The model under review builds one solid part; all positions refer to its coordinate system, in mm. A direction names the side the tool comes from. Give positions to 0.01 mm unless a question says otherwise; leave off trailing zeros. Order: outer loops, then holes, each group sorted by start corner. A loop starts at its lowest first (then second) coordinate and runs counter-clockwise, first axis right, second up. Notation, with made-up numbers: (70, 62) -> (98, 62) arc R19 cw to (98, 87) -> close; hole circle Ø2 at (11.25, 22.25). An arc over 180 degrees is marked (long way). Answer as a JSON object with one key per item and string values. Group by question number.
from build123d import *

# Parameters (mm, degrees)
SKETCH_R        = 2.6
PAD_DEPTH       = 12
SKETCH001_W     = 20
SKETCH001_H     = 20
POCKET_DEPTH    = 5
SKETCH002_R     = 4.5
POCKET001_DEPTH = 12
SKETCH003_R     = 10.85
POCKET002_DEPTH = 8
SKETCH004_R     = 5.95
POCKET003_DEPTH = 4
SKETCH005_R     = 1.5
POCKET004_DEPTH = 19
SKETCH006_R     = 2.811214
POCKET005_DEPTH = 4
SKETCH007_R     = 4
POCKET006_DEPTH = 3
SKETCH008_R     = 1.5
POCKET007_DEPTH = 16
SKETCH009_R     = 1.5
POCKET008_DEPTH = 16


with BuildPart() as part:
    # Sketch → Pad (new body)
    with BuildSketch(Plane.XY):
        with BuildLine():
            Line((-57.237457, 55.978201), (32.762543, 55.978201))
            Line((32.762543, 55.978201), (32.762543, 25.978201))
            Line((32.762543, 25.978201), (35.725993, 25.978201))
            ThreePointArc((37.762543, 23.941651), (37.166051, 25.381709), (35.725993, 25.978201))
            Line((37.762543, 23.941651), (37.762543, 20.978201))
            Line((37.762543, -6.948806), (37.762543, 20.978201))
            Line((8.727398, -6.948806), (37.762543, -6.948806))
            ThreePointArc((6.368817, -5.446224), (7.329126, -6.541247), (8.727398, -6.948806))
            Line((-1.496911, 11.421883), (6.368817, -5.446224))
            ThreePointArc((-1.496911, 11.421883), (-2.47295, 12.534842), (-3.894125, 12.949077))
            Line((-20.852174, 12.949077), (-3.894125, 12.949077))
            ThreePointArc((-20.852174, 12.949077), (-22.12751, 12.577351), (-23.003388, 11.578602))
            Line((-31.391573, -6.409918), (-23.003388, 11.578602))
            ThreePointArc((-32.237457, -6.948806), (-31.73598, -6.802638), (-31.391573, -6.409918))
            Line((-62.237457, -6.948806), (-32.237457, -6.948806))
            Line((-62.237457, 17.407665), (-62.237457, -6.948806))
            Line((-62.237457, 17.407665), (-62.237457, 24.590235))
            ThreePointArc((-60.849491, 25.978201), (-61.830931, 25.571675), (-62.237457, 24.590235))
            Line((-60.849491, 25.978201), (-57.237457, 25.978201))
            Line((-57.237457, 25.978201), (-57.237457, 55.978201))
        make_face()
        with Locations((-49.737457, 6.02373)):
            Circle(SKETCH_R, mode=Mode.SUBTRACT)
        with Locations((-31.737457, 6.02373)):
            Circle(SKETCH_R, mode=Mode.SUBTRACT)
        with Locations((25.262543, 5.551194)):
            Circle(SKETCH_R, mode=Mode.SUBTRACT)
        with Locations((7.262543, 5.551194)):
            Circle(SKETCH_R, mode=Mode.SUBTRACT)
    extrude(amount=PAD_DEPTH)

    # Sketch001 (on Face26 of Pad) → Pocket (cut)
    with BuildSketch(Plane.XY.offset(12)):
        with Locations((-49.737457, 6.02373)):
            Rectangle(SKETCH001_W, SKETCH001_H)
        with Locations((25.262543, 5.551194)):
            Rectangle(SKETCH001_W, SKETCH001_H)
    extrude(amount=-POCKET_DEPTH, mode=Mode.SUBTRACT)

    # Sketch002 (on Face5 of Pocket) → Pocket001 (cut)
    with BuildSketch(Plane.XY.offset(12)):
        with Locations((-12.237457, 40.978201)):
            Circle(SKETCH002_R)
    extrude(amount=-POCKET001_DEPTH, mode=Mode.SUBTRACT)

    # Sketch003 (on Face5 of Pocket001) → Pocket002 (cut)
    with BuildSketch(Plane.XY.offset(12)):
        with Locations((-12.237457, 40.978201)):
            Circle(SKETCH003_R)
    extrude(amount=-POCKET002_DEPTH, mode=Mode.SUBTRACT)

    # Sketch004 (on Face5 of Pocket002) → Pocket003 (cut)
    with BuildSketch(Plane.XY.offset(12)):
        with Locations((-36.737457, 40.978201)):
            Circle(SKETCH004_R)
        with Locations((12.262543, 40.978201)):
            Circle(SKETCH004_R)
    extrude(amount=-POCKET003_DEPTH, mode=Mode.SUBTRACT)

    # Sketch005 (on Face18 of Pocket003) → Pocket004 (cut)
    with BuildSketch(Plane.XZ.offset(-12.949077)):
        with Locations((-12.237457, 8)):
            Circle(SKETCH005_R)
    extrude(amount=-POCKET004_DEPTH, mode=Mode.SUBTRACT)

    # Sketch006 (on Face18 of Pocket004) → Pocket005 (cut)
    with BuildSketch(Plane.XZ.offset(-12.949077)):
        with Locations((-12.237457, 8)):
            Circle(SKETCH006_R)
    extrude(amount=-POCKET005_DEPTH, mode=Mode.SUBTRACT)

    # Sketch007 (on Face4 of Pocket005) → Pocket006 (cut)
    with BuildSketch(Plane(origin=(0, 0, 0), x_dir=(1, 0, 0), z_dir=(0, 0, -1))):
        with Locations((-49.737457, -6.02373)):
            Circle(SKETCH007_R)
        with Locations((-31.737457, -6.02373)):
            Circle(SKETCH007_R)
        with Locations((7.262543, -5.551194)):
            Circle(SKETCH007_R)
        with Locations((25.262543, -5.551194)):
            Circle(SKETCH007_R)
    extrude(amount=-POCKET006_DEPTH, mode=Mode.SUBTRACT)

    # Sketch008 (on Face9 of Pocket006) → Pocket007 (cut)
    with BuildSketch(Plane.YZ.offset(32.762543)):
        with Locations((40.978201, 10)):
            Circle(SKETCH008_R)
    extrude(amount=-POCKET007_DEPTH, mode=Mode.SUBTRACT)

    # Sketch009 (on Face3 of Pocket007) → Pocket008 (cut)
    with BuildSketch(Plane(origin=(-57.237457, 0, 0), x_dir=(0, -1, 0), z_dir=(-1, 0, 0))):
        with Locations((-40.978201, 10)):
            Circle(SKETCH009_R)
    extrude(amount=-POCKET008_DEPTH, mode=Mode.SUBTRACT)


solid = part.part
1. Take a section at A-A on x = 25. Give the boundary of the cut face in (y, z), plus the area to 3 significant figures.
2. Machinability: for faces 3 (the flat face through (27, 8, 7)), 4 (the cylindrical face through (-12.847, 14.921, 5.256)), 5 (the cylindrical face through (25.495, 39.788, 9.087)), 6 (the flat face through (-32, 9, 3)), 7 (the flat face through (2.38, 3.11, 5.92)), which of the approach directions +Z, -Z, +X, -X, +Y, -Y give a long, thin tool a straight path to every point of the face, cutting with its end or side? Answer none if there is none.
3. Take a section at D-D on y = 32. Give the boundary of the cut face in (x, z).
4. Take a section at B-B on y = 14.5. Give the boundary of the cut face in (x, z), plus the area to 3 significant figures.
5. Take a section at C-C on x = 7.5. Give the boundary of the cut face in (y, z), plus the area to 3 significant figures.
6. Draft analysis for pull direction X (two halves, no side actions). For faces 1 (the cylindrical face through (3.266, 5.375, 1.479)), 2 (the cylindrical face through (-49.97, 39.547, 10.451)), state which applies: pulls with the +X half, pulls with the -X half, needs draft (parallel to the pull), parting line crosses it, or undercut.
7. For pin 1 (9 mm diameter, centred on x = -49.74, y = 6.02, fed in from +Z); pin 2 (3 mm diameter, centred on x = -13, z = 6, fed in from -Y); pin 3 (4 mm diameter, centred on y = 40.5, z = 5.5, fed in from +X), all flat-tipped, find the tip position at first contact; note any pin that passes through.
8. For probe 1 along Y at (x, z) = (-47.5, 10); probe 2 along X at (y, z) = (12, 10.25); probe 3 along Y at (x, z) = (-45.5, 10.5), list the stretches that pass through material, from the lowest coordinate up. Write a range as [from, to].
Checks:
{
 "1": {"outline": "(-6.95, 0) -> (1.56, 0) -> (1.56, 3) -> (2.96, 3) -> (2.96, 7) -> (-4.45, 7) -> (-4.45, 12) -> (-6.95, 12) -> close; (8.14, 3) -> (9.54, 3) -> (9.54, 0) -> (55.98, 0) -> (55.98, 12) -> (15.55, 12) -> (15.55, 7) -> (8.14, 7) -> close; hole circle Ø3 at (40.98, 10)", "area": "603 mm2"},
 "2": {"face 3": "+Z", "face 4": "-Y", "face 5": "+X", "face 6": "-Z", "face 7": "+Z, -Z, -Y"},
 "3": {"outline": "(-57.24, 0) -> (32.76, 0) -> (32.76, 12) -> (-6.15, 12) -> (-6.15, 4) -> (-18.33, 4) -> (-18.33, 12) -> (-57.24, 12) -> close"},
 "4": {"outline": "(-62.24, 0) -> (37.76, 0) -> (37.76, 12) -> (35.26, 12) -> (35.26, 7) -> (15.26, 7) -> (15.26, 12) -> (-39.74, 12) -> (-39.74, 7) -> (-59.74, 7) -> (-59.74, 12) -> (-62.24, 12) -> close; hole circle Ø5.62 at (-12.24, 8)", "area": "975 mm2"},
 "5": {"outline": "(-6.64, 0) -> (1.56, 0) -> (1.56, 3) -> (2.96, 3) -> (2.96, 12) -> (-6.64, 12) -> close; (8.14, 3) -> (9.54, 3) -> (9.54, 0) -> (55.98, 0) -> (55.98, 12) -> (44.54, 12) -> (44.54, 8) -> (37.41, 8) -> (37.41, 12) -> (8.14, 12) -> close", "area": "652 mm2"},
 "6": {"face 1": "undercut", "face 2": "needs draft"},
 "7": {"pin 1": "stops at z = 7", "pin 2": "stops at y = 12.95", "pin 3": "stops at x = 32.76"},
 "8": {"probe 1": "y = [-6.95, -3.98], [16.02, 39.48], [42.48, 55.98]", "probe 2": "x = [-62.24, -59.74], [-39.74, -22.75], [-1.86, 15.26], [35.26, 37.76]", "probe 3": "y = [-6.95, -3.98], [16.02, 39.56], [42.39, 55.98]"}
}
